Model file for the job. Use its own axes, mm. Face numbers are marked on the shaded views. Round coordinates to 2 decimals unless told otherwise and drop trailing zeros. Loops run counter-clockwise (first coordinate to the right, second up) from the corner with the lowest first, then second, coordinate; pieces in that order, holes last. Notation, with made-up numbers: (-24.75, -0.5) - (10.25, -0.5) arc R8 ccw to (10.25, 3.5) - close; hole circle Ø8 at (34.25, 5). An arc over 180 degrees is marked (long way). Answer as a JSON object with one key per item and string values.
from build123d import *

# Parameters (mm, degrees)
EXTRUDE_1_DEPTH      = 150
SKETCH_3_W           = 134.939871442
SKETCH_3_H           = 65.077722632
SKETCH_3_W_2         = 12.852713976
SKETCH_3_H_2         = 65.21229221
SKETCH_3_W_3         = 22.325721816
CUT_EXTRUDE_5_DEPTH  = 100
SKETCH_4_R           = 10
CUT_EXTRUDE_6_DEPTH  = 100
CUT_EXTRUDE_7_DEPTH  = 542.338297497
SKETCH_9_W           = 120
SKETCH_9_H           = 50
EXTRUDE_5_DEPTH      = 200
SKETCH_12_W          = 124.1848091
SKETCH_12_H          = 30
CUT_EXTRUDE_14_DEPTH = 60
SKETCH_13_R          = 15
CUT_EXTRUDE_15_DEPTH = 459.970793946
CUT_EXTRUDE_16_DEPTH = 600
CUT_EXTRUDE_18_DEPTH = 600
CUT_EXTRUDE_23_DEPTH = 600


with BuildPart() as part:
    # 草图1 → 凸台-拉伸1 (new body)
    with BuildSketch(Plane(origin=(0, 0, 0), x_dir=(1, 0, 0), z_dir=(0, 1, 0))):
        Polygon((-296.625222025, 119.18294849), (103.374777975, 114.564831261), (393.424758435, -189.19660282), (363.661240814, -189.19660282), (83.221819158, 38.873627041), (-316.778180842, -14.24353747), align=None)
    extrude(amount=EXTRUDE_1_DEPTH)

    # 草图3 → 切除-拉伸5 (cut)
    with BuildSketch(Plane(origin=(-307.609145788, 0, -46.461798062), x_dir=(-0.14934769539615667, 0, 0.9887847419331757), z_dir=(-0.9887847419331757, 0, -0.14934769539615664))):
        Polygon((-73.54598766, 84.922277368), (-73.54598766, 150), (-110.299587537, 150), (-108.970561803, 84.922277368), align=None)
        with Locations((-6.076051939, 117.461138684)):
            Rectangle(SKETCH_3_W, SKETCH_3_H)
        with Locations((67.82024077, 117.461138684)):
            Rectangle(SKETCH_3_W_2, SKETCH_3_H)
        Polygon((-73.54598766, 0), (-73.54598766, 65.21229221), (-88.627784697, 65.21229221), (-110.299587537, 65.21229221), (-110.299587537, 0), align=None)
        with Locations((-6.076051939, 32.606146105)):
            Rectangle(SKETCH_3_W, SKETCH_3_H_2)
        with Locations((72.55674469, 32.606146105)):
            Rectangle(SKETCH_3_W_3, SKETCH_3_H_2)
    extrude(amount=-CUT_EXTRUDE_5_DEPTH, mode=Mode.SUBTRACT)

    # 草图4 → 切除-拉伸6 (cut)
    with BuildSketch(Plane(origin=(0, 84.922277368, 0), x_dir=(1, 0, 0), z_dir=(0, 1, 0))):
        with Locations(Location((-255.193452216, 58.700607885, 0), (0, 0, 270))):
            Circle(SKETCH_4_R)
    extrude(amount=-CUT_EXTRUDE_6_DEPTH, mode=Mode.SUBTRACT)

    # 草图5 → 切除-拉伸7 (cut, through all)
    with BuildSketch(Plane(origin=(111.294466259, 0, -106.270757713), x_dir=(-0.6905951915709648, 0, -0.7232415097179243), z_dir=(0.7232415097179243, 0, -0.6905951915709648))):
        Polygon((11.467916923, 150), (-408.532083077, 100), (-408.532083077, 150), align=None)
        Polygon((11.467916923, 0), (-408.532083077, 50), (-408.532083077, 0), align=None)
    extrude(amount=-CUT_EXTRUDE_7_DEPTH, mode=Mode.SUBTRACT)

    # 草图9 → 凸台-拉伸5 (add)
    with BuildSketch(Plane(origin=(-3.630590426, 0, -27.340242721), x_dir=(0.9912979424923631, 0, -0.13163733972702288), z_dir=(0.13163733972702288, 0, 0.9912979424923631))):
        with Locations((-146.786325955, 75)):
            Rectangle(SKETCH_9_W, SKETCH_9_H)
    extrude(amount=-EXTRUDE_5_DEPTH)

    # 草图12 → 切除-拉伸14 (cut)
    with BuildSketch(Plane(origin=(-29.958058371, 0, -225.599831219), x_dir=(-0.991297942492363, 0, 0.1316373397270229), z_dir=(-0.1316373397270229, 0, -0.991297942492363))):
        with Locations((145.743983676, 75)):
            Rectangle(SKETCH_12_W, SKETCH_12_H)
    extrude(amount=-CUT_EXTRUDE_14_DEPTH, mode=Mode.SUBTRACT)

    # 草图13 → 切除-拉伸15 (cut, through all)
    with BuildSketch(Plane(origin=(0, 50, 0), x_dir=(-1, 0, 0), z_dir=(0, -1, 0))):
        with Locations(Location((170.201547688, 166.625352062, 0), (0, 0, 270))):
            Circle(SKETCH_13_R)
    extrude(amount=-CUT_EXTRUDE_15_DEPTH, mode=Mode.SUBTRACT)

    # 草图14 → 切除-拉伸16 (cut)
    with BuildSketch(Plane.XZ.offset(-65.21229221)):
        with BuildLine():
            Line((-316.778180842, 14.24353747), (-213.573939594, 0.538745819))
            ThreePointArc((-213.573939594, 0.538745819), (-264.946374334, -9.940662831), (-308.780384447, -38.707390387))
            Line((-308.780384447, -38.707390387), (-316.778180842, 14.24353747))
        make_face()
    extrude(amount=-CUT_EXTRUDE_16_DEPTH, mode=Mode.SUBTRACT)

    # 草图15 → 切除-拉伸18 (cut)
    with BuildSketch(Plane(origin=(0, 65.21229221, 0), x_dir=(-1, 0, 0), z_dir=(0, -1, 0))):
        with BuildLine():
            ThreePointArc((245.824298176, 118.596436936), (278.450621549, 106.430151008), (302.373134739, 81.127802248))
            Line((302.373134739, 81.127802248), (296.625222025, 119.18294849))
            Line((296.625222025, 119.18294849), (245.824298176, 118.596436936))
        make_face()
    extrude(amount=-CUT_EXTRUDE_18_DEPTH, mode=Mode.SUBTRACT)

    # 草图16 → 切除-拉伸23 (cut)
    with BuildSketch(Plane(origin=(0, 65.21229221, 0), x_dir=(-1, 0, 0), z_dir=(0, -1, 0))):
        with BuildLine():
            Line((291.65867542, 24.560550225), (320.979664595, 36.581658237))
            Line((320.979664595, 36.581658237), (321.34512954, 76.765505909))
            Line((321.34512954, 76.765505909), (299.707915755, 85.363339544))
            ThreePointArc((299.707915755, 85.363339544), (302.777897257, 54.022742019), (291.65867542, 24.560550225))
        make_face()
    extrude(amount=-CUT_EXTRUDE_23_DEPTH, mode=Mode.SUBTRACT)


solid = part.part
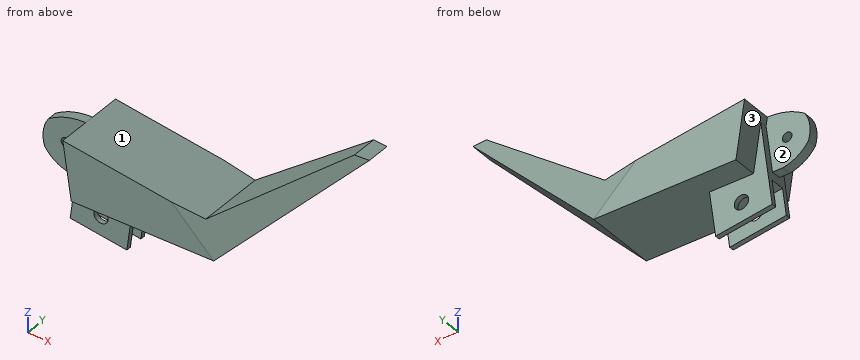
1) Slice it at C-C on x = 64. List the corners of the cut face in (y, z).
Values follow:
{"outline": "(0, -115.02) - (150, -115.02) - (150, -76.97) - (146.5, -36.32) - (3.5, -36.32) - (0, -76.97) - close"}
2) Probe probe 1 along Y at (x, z) = (-173, -196); probe 2 along Y at (x, z) = (-239, -86); probe 3 along X at (y, z) = (66, -64.5). List the from-to ranges inside material, lowest first.
Values follow:
{"probe 1": "50 to 60, 90 to 100", "probe 2": "65.21 to 84.92", "probe 3": "-303.36 to -263.34, -247.05 to 151.18"}
3) Slice it at D-D on y = 27.5. List the corners of the cut face in (x, z).
Values follow:
{"outline": "(-213.57, 0.54) - (-195.67, -118.02) - (103.37, -114.56) - (262.9, 52.5) - (231.94, 82.07) - (83.22, -38.87) - close"}
4) Slice it at B-B on z = -101. List the corners of the cut face in (x, y), then the cut area to 3 significant figures.
Values follow:
{"outline": "(-285.68, 65.21) - (-222.01, 65.21) - (-222.01, 50) - (-198.24, 50) - (-198.24, 0) - (89.17, 0) - (116.33, 2.23) - (116.33, 147.77) - (89.17, 150) - (-198.24, 150) - (-198.24, 100) - (-222.01, 100) - (-222.01, 84.92) - (-285.68, 84.92) - close", "area": "49,600 mm²"}
5) Slice it at A-A on z = -6.5. List the corners of the cut face in (x, y), then the cut area to 3 significant figures.
Values follow:
{"outline": "(-255.68, 65.21) - (-212.51, 65.21) - (-212.51, 0) - (-160.57, 0) - (-160.57, 150) - (-212.51, 150) - (-212.51, 84.92) - (-255.68, 84.92) - close; (123.03, 10.92) - (206.56, 17.79) - (206.56, 132.21) - (123.03, 139.08) - close", "area": "18,800 mm²"}
6) Two-plate mould, pull along X, no slides. Class the marked faces 1, 2 and 3: pulls with the +X half, pulls with the -X half, needs draft (parallel to the pull), parting line crosses it, or undercut.
Values follow:
{"face 1": "undercut", "face 2": "needs draft", "face 3": "pulls with the -X half"}
7) Drop flat-ended pins along their axis: P1, Ø2, axis at x = 230.5, y = 105, coming from the +Z side; P2, Ø1, axis at x = 58, y = 86, coming from the -Z side; P3, Ø4, axis at y = 86, z = -38.5, coming from the -X side; P4, Ø24, axis at x = -170.2, z = -166.63, coming from the -Y side. Give the stop position or say it passes through.
Values follow:
{"P1": "z = 81.72", "P2": "z = -115.09", "P3": "x = -299.47", "P4": "through"}
